Geometry: see drawing. Coordinates: mm, zero at the bounding-box minimum. Give positions to 0.01 mm unless a question says otherwise; leave off trailing zeros. Order: outer loops, then holes, each group sorted by start corner. A loop starts at its lowest first (then second) coordinate and runs counter-clockwise, first axis right, second up. Notation, with made-up numbers: M -24.5,-24 L 14.5,-24 A19 ccw 14.5,-9 Z; hole C 68.5,61 d10. An arc over 180 degrees is marked long. Use a Markdown table: item, result.
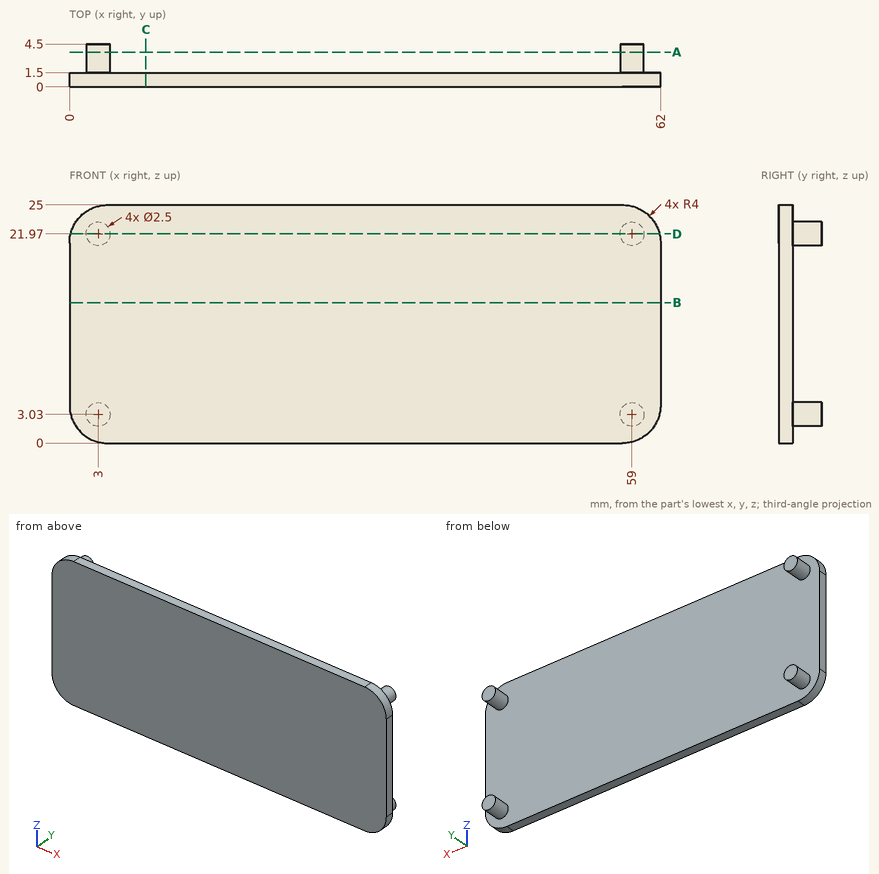
1) Material intervals for line 1 (Y direction, x = 11, z = 22.75); line 2 (X direction, y = 1.7, z = 23); line 3 (X direction, y = 1.8, z = 2.5), sorted ascending. Write a range as from..to.
Response values:
| item | result |
|---|---|
| line 1 | y = 0..1.5 |
| line 2 | x = 2.29..3.71, 58.29..59.71 |
| line 3 | x = 1.87..4.13, 57.87..60.13 |
2) Cut plane C-C on x = 8. Return loops of the section in (y, z), and give its area (3 significant figures).
Response values:
| item | result |
|---|---|
| outline | M 0,0 L 1.5,0 L 1.5,25 L 0,25 Z |
| area | 37.5 mm² |
3) Cut plane B-B on z = 14.75. Return loops of the section in (x, y).
Response values:
| item | result |
|---|---|
| outline | M 0,0 L 62,0 L 62,1.5 L 0,1.5 Z |
4) Cut plane A-A on y = 3.65. Return loops of the section in (x, z).
Response values:
| item | result |
|---|---|
| outline | C 3,3.03 d2.5; C 3,21.97 d2.5; C 59,3.03 d2.5; C 59,21.97 d2.5 |
5) First-contact query: pin 1 Ø12.5 at (x, z) = (42.5, 15.5) entering from +Y. Flat tip, straight axial feed; report the tip coordinate or a pass-through.
Response values:
| item | result |
|---|---|
| pin 1 | stops at y = 1.5 |
6) Cut plane D-D on z = 21.97. Return loops of the section in (x, y), and give its area (3 significant figures).
Response values:
| item | result |
|---|---|
| outline | M 0.12,0 L 61.88,0 L 61.88,1.5 L 60.25,1.5 L 60.25,4.5 L 57.75,4.5 L 57.75,1.5 L 4.25,1.5 L 4.25,4.5 L 1.75,4.5 L 1.75,1.5 L 0.12,1.5 Z |
| area | 108 mm² |
